Source: CAD feature listing. Evaluate the final solid. Frame: model axes, mm. Face numbers are marked on the shaded views. A direction names the side the tool comes from. Round coordinates to 2 decimals unless told otherwise and drop trailing zeros. Order: outer loops, then holes, each group sorted by start corner. A loop starts at its lowest first (then second) coordinate and runs counter-clockwise, first axis right, second up. Notation, with made-up numbers: (25, 33) - (48, 33) arc R18 ccw to (48, 45) - close; hole circle Ø4 at (16.25, 6.25). An arc over 180 degrees is marked (long way). Return JSON: item names as keys, results as strings. Group by question number.
1) Section D-D, the plane y = 1.75. Return loops of the section in (x, z).
2) Ray query, line 1 (Y direction, x = 3.25, z = 9.25); line 2 (Z direction, x = 2.5, y = 5). Return the intervals inside material, ascending. Write a range as from..to.
3) Section C-C, the plane z = 3.75. Return loops of the section in (x, y), plus the area to 3 significant figures.
4) Access query for the marked faces 1, 2, 3 and 4. Directions: +Z, -Z, +X, -X, +Y, -Y. A direction counts if a zero-diameter tool reaches every point of the face in a straight line with its end or side. Return the directions, or none.
5) Contact query for flat-ended pins moving along their axis: P1, Ø4.5, axis at x = -2, y = 4.5, coming from the -Z side; P2, Ø4, axis at x = -7.5, z = 2, coming from the +Y side; P3, Ø1.2, axis at y = 4.5, z = 1, coming from the -X side. Output: stop coordinate, or through.
6) Section B-B, the plane x = 4.75. Return loops of the section in (y, z), plus the area to 3 significant figures.
7) Section A-A, the plane y = 3.75. Return loops of the section in (x, z).
```python
from build123d import *

# Parameters (mm, degrees)
SKETCH1_W           = 20
SKETCH1_H           = 20
BOSS_EXTRUDE1_DEPTH = 1
FILLET2_R           = 5
BOSS_EXTRUDE3_DEPTH = 8
CHAMFER1_SIZE       = 2
CHAMFER3_SIZE       = 2


with BuildPart() as part:
    # Sketch1 → Boss-Extrude1 (new body)
    with BuildSketch(Plane(origin=(0, 0, 0), x_dir=(1, 0, 0), z_dir=(0, 1, 0))):
        Rectangle(SKETCH1_W, SKETCH1_H)
    extrude(amount=BOSS_EXTRUDE1_DEPTH)

    # Fillet2
    fillet2_edges = [part.edges().sort_by_distance(p)[0] for p in [
        (10, 0.5, 10),
        (-10, 0.5, 10),
        (-10, 0.5, -10),
        (10, 0.5, -10),
    ]]
    fillet(fillet2_edges, radius=FILLET2_R)

    # Sketch3 → Boss-Extrude3 (add)
    with BuildSketch(Plane(origin=(0, 1, 0), x_dir=(1, 0, 0), z_dir=(0, 1, 0))):
        with BuildLine():
            Line((-7, 5), (-7, -5))
            ThreePointArc((-7, -5), (-6.414213562, -6.414213562), (-5, -7))
            Line((-5, -7), (5, -7))
            ThreePointArc((5, -7), (6.414213562, -6.414213562), (7, -5))
            Line((7, -5), (7, 5))
            ThreePointArc((7, 5), (6.414213562, 6.414213562), (5, 7))
            Line((5, 7), (-5, 7))
            ThreePointArc((-5, 7), (-6.414213562, 6.414213562), (-7, 5))
        make_face()
    extrude(amount=BOSS_EXTRUDE3_DEPTH)

    # Chamfer1
    chamfer1_edges = [part.edges().sort_by_distance(p)[0] for p in [
        (-6.414213562, 1, -6.414213562),
        (-7, 1, 0),
        (-6.414213562, 1, 6.414213562),
        (0, 1, 7),
        (6.414213562, 1, 6.414213562),
        (7, 1, 0),
        (6.414213562, 1, -6.414213562),
        (0, 1, -7),
    ]]
    chamfer(chamfer1_edges, length=CHAMFER1_SIZE)

    # Chamfer3
    chamfer3_edges = [part.edges().sort_by_distance(p)[0] for p in [
        (-6.414213562, 9, -6.414213562),
        (-7, 9, 0),
        (-6.414213562, 9, 6.414213562),
        (0, 9, 7),
        (6.414213562, 9, 6.414213562),
        (7, 9, 0),
        (6.414213562, 9, -6.414213562),
        (0, 9, -7),
    ]]
    chamfer(chamfer3_edges, length=CHAMFER3_SIZE - 0.0001)  # a hair under: the kernel refuses the full size


solid = part.part
```
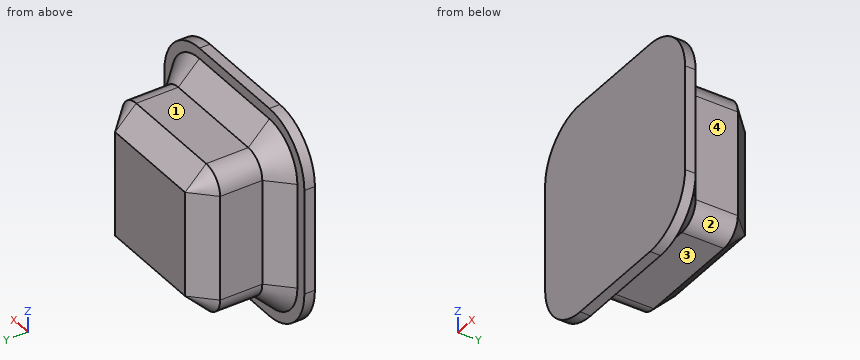
Geometry check:
{
 "1": {"outline": "(-8.25, -5) arc R3.25 ccw to (-5, -8.25) - (5, -8.25) arc R3.25 ccw to (8.25, -5) - (8.25, 5) arc R3.25 ccw to (5, 8.25) - (-5, 8.25) arc R3.25 ccw to (-8.25, 5) - close"},
 "2": {"line 1": "0..1", "line 2": "-7..7"},
 "3": {"outline": "(-10, 0) - (10, 0) - (10, 1) - (9, 1) - (7, 3) - (7, 7) - (5, 9) - (-5, 9) - (-7, 7) - (-7, 3) - (-9, 1) - (-10, 1) - close", "area": "132 mm2"},
 "4": {"face 1": "+Z, +X, -X, +Y", "face 2": "-Z, +X, +Y", "face 3": "-Z, +X, -X, +Y", "face 4": "+Z, -Z, +X, +Y"},
 "5": {"P1": "z = -7.75", "P2": "y = 8.5", "P3": "x = -7"},
 "6": {"outline": "(0, -10) - (1, -10) - (1, -9) - (3, -7) - (7, -7) - (9, -5) - (9, 5) - (7, 7) - (3, 7) - (1, 9) - (1, 10) - (0, 10) - close", "area": "132 mm2"},
 "7": {"outline": "(-7, -5) arc R2 ccw to (-5, -7) - (5, -7) arc R2 ccw to (7, -5) - (7, 5) arc R2 ccw to (5, 7) - (-5, 7) arc R2 ccw to (-7, 5) - close"}
}
